Autodesk Inventor part; units mm, degrees
ref_plane "YZ Plane" through (0, 0, 0) normal (1, 0, 0) x (0, 1, 0)
ref_plane "XZ Plane" through (0, 0, 0) normal (0, 1, 0) x (-1, 0, 0)
ref_plane "XY Plane" through (0, 0, 0) normal (0, 0, 1) x (1, 0, 0)
sketch "Sketch1" plane through (0, 0, 0) normal (0, 0, 1) x (1, 0, 0)
  circle A0 centre (0, 0) radius 21
  circle A1 centre (200, 0) radius 15
  line L0 (0, 0) -> (200, 0)
  line L1 (0.6307, 20.9905) -> (200.45, 14.9932)
  line L2 (0.6307, -20.9905) -> (200.45, -14.9932)
  dimension "d10" = 15
  dimension "d11" = 21
  dimension "d9" = 200
extrude "Extrusion1" add sketch "Sketch1" along normal blind 6
sketch "Sketch2" plane through (0, 0, 6) normal (0, 0, 1) x (1, 0, 0)
  circle A0 centre (0, 0) radius 1.75
  arc A1 (200.45, -14.9932) -> (200.45, 14.9932) centre (200, 0) ccw
  circle A2 centre (200, 0) radius 1.75
  point P0 (293.3543, -13.4475)
  point P1 (293.3543, 13.4475)
  point P2 (250.3596, -14.9957)
  point P3 (250.3596, 14.9957)
  dimension "d5" = 3.5
  dimension "d6" = 3.5
extrude "Extrusion2" cut sketch "Sketch2" against normal through all
properties part number "Tibia"
Geometry check sheet. Reference: the model listing, model coordinates, mm. Give positions to 0.01 mm unless a question says otherwise; leave off trailing zeros. Loops run counter-clockwise (first coordinate to the right, second up) from the corner with the lowest first, then second, coordinate; pieces in that order, holes last. Notation, with made-up numbers: M 33,63 L 39,63 A31 ccw 39,88 Z; hole C 63.25,-29 d1. An arc over 180 degrees is marked long. Answer as a JSON object with one key per item and string values. Group by question number.
Item 1: Gauge pin test, flat ends, axial feed: pin 1 (2 mm diameter, centred on y = 7.5, z = 3.5, fed in from +X); pin 2 (3 mm diameter, centred on x = 200, y = 0, fed in from -Z). Record the tip position at first contact, or that the pin passes through.
Item 2: Sectioned sample at C-C on x = 53.5. Record the boundary of the cut face in (y, z), plus the area to 3 significant figures.
Item 3: Material ranges on L1, parallel to Y at x = 200, z = 4.2; L2, parallel to X at y = -0.5, z = 1; L3, parallel to Y at x = 0, z = 4.55, recorded low to high.
Item 4: Sectioned sample at B-B on x = 145.5. Record the boundary of the cut face in (y, z).
Item 5: Sectioned sample at A-A on z = 3.3. Record the boundary of the cut face in (x, y), plus the area to 3 significant figures.
Findings below:
{
 "1": {"pin 1": "x = 213.52", "pin 2": "through"},
 "2": {"outline": "M -19.4,0 L 19.4,0 L 19.4,6 L -19.4,6 Z", "area": "233 mm2"},
 "3": {"L1": "-15.01 to -1.75, 1.75 to 15.01", "L2": "-20.99 to -1.68, 1.68 to 198.32, 201.68 to 214.99", "L3": "-21 to -1.75, 1.75 to 21"},
 "4": {"outline": "M -16.64,0 L 16.64,0 L 16.64,6 L -16.64,6 Z"},
 "5": {"outline": "M 0.63,-20.99 L 200.45,-14.99 A15 ccw 200.45,14.99 L 0.63,20.99 A21 ccw long Z; hole C 0,0 d3.5; hole C 200,0 d3.5", "area": "8,230 mm2"}
}
